Geometry check sheet. Reference: the model listing, model coordinates, mm. A direction names the side the tool comes from. Give positions to 0.01 mm unless a question says otherwise; leave off trailing zeros. Write each loop counter-clockwise with the first axis right and the second up, starting at its lowest first coordinate (ties: lowest second). Pieces come first, ordered by that corner, then holes. Notation, with made-up numbers: M 25.25,-4.75 L 76.25,-4.75 A22 ccw 76.25,22.25 Z; hole C 10.5,84 d11. An arc over 180 degrees is marked long. One line per item, written item: value. Start each with the question number.
1. Release check for a two-part mould opening along Z. For faces 3 (the face through (-2, 28.4, -4)), 4 (the face through (-2.87, 27.32, 2.64)), 5 (the face through (0.96, 6.58, 0.3)) record: pulls with the +Z half, pulls with the -Z half, needs draft (parallel to the pull), parting line crosses it, or undercut.
2. Cross-section at A-A on z = 0. Record the cut outline in (x, y) (3 decimals), then the cut area to 3 significant figures.
3. Scan lines: line 1 (Z direction, x = 0, y = 17.5) (3 decimals); line 2 (Z direction, x = -0.75, y = 21.5); line 3 (Z direction, x = -2.25, y = 14.5). Record each from-to range of solid material in increasing order.
4. Gauge pin test, flat ends, axial feed: pin 1 (4 mm diameter, centred on x = 4, y = 20.5, fed in from -Z); pin 2 (3 mm diameter, centred on x = -2, z = 0.5, fed in from -Y); pin 3 (3 mm diameter, centred on y = 21.5, z = 3, fed in from +X); pin 4 (5 mm diameter, centred on y = 20.5, z = 4.5, fed in from -X). Record the tip position at first contact, or that the pin passes through.
5. Cross-section at C-C on y = 29.5. Record the cut outline in (x, z) (3 decimals).
6. Cross-section at D-D on y = 21. Record the cut outline in (x, z) (3 decimals).
7. Tool access check on faces 1 (the face through (-4.5, 12.4, -3.5)), 2 (the face through (-1.22, 20.86, -0.93)). Record the directions out of +Z, -Z, +X, -X, +Y, -Y that give a thin tool (end or side, any length) a straight path to the whole face; none if there is none.
8. Cross-section at B-B on x = 0. Record the cut outline in (y, z) (3 decimals), then the cut area to 3 significant figures.
from build123d import *


with BuildPart() as part:
    # Sketch2 → Revolve1 (revolve)
    with BuildSketch(Plane.XY):
        with BuildLine():
            Line((0, 0), (5.7, 0))
            Line((5.7, 0), (5.7, 24.4))
            ThreePointArc((5.7, 24.4), (5.172792206, 25.672792206), (3.9, 26.2))
            Line((3.9, 26.2), (3.9, 28.4))
            Line((3.9, 28.4), (5.4, 28.4))
            Line((5.4, 28.4), (5.4, 32.2))
            Line((5.4, 32.2), (1.535, 32.2))
            Line((1.535, 32.2), (1.535, 9.834154564))
            Line((1.535, 9.834154564), (0.493536823, 3.419866334))
            ThreePointArc((0.493536823, 3.419866334), (0.323985468, 3.119167469), (0, 3))
            Line((0, 3), (0, 0))
        make_face()
    revolve(axis=Axis((0, 32.2, 0), (0, -1, 0)))


solid = part.part
Report:
1. face 3: needs draft
1. face 4: parting line crosses it
1. face 5: undercut
2. outline: M -5.7,0 L 5.7,0 L 5.7,24.4 A1.8 ccw 3.9,26.2 L 3.9,28.4 L 5.4,28.4 L 5.4,32.2 L 1.535,32.2 L 1.535,9.834 L 0.494,3.42 A0.5 cw -0.494,3.42 L -1.535,9.834 L -1.535,32.2 L -5.4,32.2 L -5.4,28.4 L -3.9,28.4 L -3.9,26.2 A1.8 ccw -5.7,24.4 Z
2. area: 274 mm^2
3. line 1: z = -5.7 to -1.535, 1.535 to 5.7
3. line 2: z = -5.65 to -1.34, 1.34 to 5.65
3. line 3: z = -5.24 to 5.24
4. pin 1: stops at z = -5.34
4. pin 2: stops at y = 0
4. pin 3: stops at x = 5.5
4. pin 4: stops at x = -5.34
5. outline: C 0,0 d10.8; hole C 0,0 d3.07
6. outline: C 0,0 d11.4; hole C 0,0 d3.07
7. face 1: +Y, -Y
7. face 2: +Y
8. outline: M 0,-5.7 L 24.4,-5.7 A1.8 ccw 26.2,-3.9 L 28.4,-3.9 L 28.4,-5.4 L 32.2,-5.4 L 32.2,-1.535 L 9.834,-1.535 L 3.42,-0.494 A0.5 cw 3.42,0.494 L 9.834,1.535 L 32.2,1.535 L 32.2,5.4 L 28.4,5.4 L 28.4,3.9 L 26.2,3.9 A1.8 ccw 24.4,5.7 L 0,5.7 Z
8. area: 274 mm^2
